Work out the finished part from the listing and answer in its coordinate system (mm). A direction names the side the tool comes from. Coordinates: 2 decimals unless noted, no trailing zeros. Loops run counter-clockwise (first coordinate to the right, second up) from the corner with the lowest first, then second, coordinate; pieces in that order, holes last.
```python
from build123d import *

# Parameters (mm, degrees)
F0_W     = 2.54
F0_H     = 2.54
F1_DEPTH = 6.35
F3_DEPTH = 2.54


# Not quite as in the source:
# - a feature names something its author has since deleted; it is built from what else it names


with BuildPart() as f1:
    # F0 (on Front) → F1 (new body)
    with BuildSketch(Plane.XZ):
        with BuildLine():
            Line((-10.8688886, 57.531), (-10.8688886, 54.991))
            ThreePointArc((-10.8688886, 54.991), (-3.183423767, 51.807576233), (0, 44.1221114))
            Line((0, 44.1221114), (0, 0))
            Line((0, 0), (2.54, 0))
            Line((2.54, 0), (2.54, 46.6621114))
            ThreePointArc((2.54, 46.6621114), (-0.643423767, 54.347576233), (-8.3288886, 57.531))
            Line((-8.3288886, 57.531), (-10.8688886, 57.531))
        make_face()
        with BuildLine():
            Line((-14.5311114, 54.991), (-10.8688886, 54.991))
            Line((-10.8688886, 54.991), (-10.8688886, 57.531))
            Line((-10.8688886, 57.531), (-17.0711114, 57.531))
            ThreePointArc((-17.0711114, 57.531), (-24.756576233, 54.347576233), (-27.94, 46.6621114))
            Line((-27.94, 46.6621114), (-27.94, 0))
            Line((-27.94, 0), (-25.4, 0))
            Line((-25.4, 0), (-25.4, 44.1221114))
            ThreePointArc((-25.4, 44.1221114), (-22.216576233, 51.807576233), (-14.5311114, 54.991))
        make_face()
        with Locations((1.27, -1.27)):
            Rectangle(F0_W, F0_H)
        with Locations((-26.67, -1.27)):
            Rectangle(F0_W, F0_H)
    extrude(amount=F1_DEPTH)

    # F2 (on Front) → F3 (join)
    with BuildSketch(Plane.XZ):
        with BuildLine():
            Line((-27.94, -2.54), (0, -2.54))
            Line((0, -2.54), (2.54, -2.54))
            Line((2.54, -2.54), (2.54, 46.6621114))
            ThreePointArc((2.54, 46.6621114), (-0.643423767, 54.347576233), (-8.3288886, 57.531))
            Line((-8.3288886, 57.531), (-17.0711114, 57.531))
            ThreePointArc((-17.0711114, 57.531), (-24.756576233, 54.347576233), (-27.94, 46.6621114))
            Line((-27.94, 46.6621114), (-27.94, -2.54))
        make_face()
    extrude(amount=F3_DEPTH)


solid = f1.part
```
1. A cutting plane is placed at A-A, the plane y = -5. Give the vertices of the cut face in (x, z), then the cut area to 3 significant figures.
2. Each of these flat-tipped pins is pushed along its axis until it touches: P1, Ø12.5, axis at x = -13.5, z = 39, coming from the -Y side; P2, Ø1.1, axis at x = -12, y = -5, coming from the -Z side. Where does it stop, or does it pass through?
3. Straight lines are drawn through the part: probe 1 along X at (y, z) = (-4, 7.5); probe 2 along Y at (x, z) = (-7, 3); probe 3 along X at (y, z) = (-6, 54). For each, find the intervals that lie inside material, in ascending order.
4. A cutting plane is placed at D-D, the plane y = -1.75. Give the vertices of the cut face in (x, z), then the cut area to 3 significant figures.
5. A cutting plane is placed at C-C, the plane x = -4. Give the vertices of the cut face in (y, z).
6. For faces 1 (the flat face through (-13, -2, -2.54)), 2 (the flat face through (-25.4, -4, 20)), determine the directions among +Z, -Z, +X, -X, +Y, -Y from which every point of the face is accessible in a straight line to the end or side of a thin tool.
7. Determine the mould class of faces 3 (the flat face through (2.54, -3, 22)), 4 (the flat face through (-27.94, -3, 22)), 5 (the cylindrical face through (-3.268, -4.418, 51.892)) for opening direction X: released by +X, released by -X, zero draft, split by the parting line, or undercut.
8. A cutting plane is placed at B-B, the plane z = 1.5. Give the vertices of the cut face in (x, y).
Answers below:
1. outline: (-27.94, -2.54) - (-25.4, -2.54) - (-25.4, 44.12) arc R10.87 cw to (-14.53, 54.99) - (-10.87, 54.99) arc R10.87 cw to (0, 44.12) - (0, -2.54) - (2.54, -2.54) - (2.54, 46.66) arc R10.87 ccw to (-8.33, 57.53) - (-17.07, 57.53) arc R10.87 ccw to (-27.94, 46.66) - close
1. area: 370 mm2
2. P1: stops at y = -2.54
2. P2: stops at z = 54.99
3. probe 1: x = -27.94 to -25.4, 0 to 2.54
3. probe 2: y = -2.54 to 0
3. probe 3: x = -25.09 to -19.07, -6.33 to -0.31
4. outline: (-27.94, -2.54) - (2.54, -2.54) - (2.54, 46.66) arc R10.87 ccw to (-8.33, 57.53) - (-17.07, 57.53) arc R10.87 ccw to (-27.94, 46.66) - close
4. area: 1,780 mm2
5. outline: (-6.35, 52.55) - (-2.54, 52.55) - (-2.54, -2.54) - (0, -2.54) - (0, 56.63) - (-6.35, 56.63) - close
6. face 1: -Z, +X, -X, +Y, -Y
6. face 2: -Z, -Y
7. face 3: released by +X
7. face 4: released by -X
7. face 5: undercut
8. outline: (-27.94, -6.35) - (-25.4, -6.35) - (-25.4, -2.54) - (0, -2.54) - (0, -6.35) - (2.54, -6.35) - (2.54, 0) - (-27.94, 0) - close
